Could you check a few things on this model? Use its own coordinates, in mm. Face numbers are marked on the shaded views. Give positions to 0.01 mm unless a question says otherwise; leave off trailing zeros. Loops run counter-clockwise (first coordinate to the right, second up) from the corner with the lowest first, then second, coordinate; pieces in that order, holes last. Notation, with made-up numbers: M 9,-23.5 L 39,-23.5 A15 ccw 39,0.5 Z; hole C -32.5,-4 d8. An arc over 180 degrees is marked long. Return JSON: item names as keys, results as strings. Group by question number.
1. If we section it at B-B (z = 25.5): Write out the boundary of the cut face in (x, y), plus the area to 3 significant figures.
2. If we mould it in two halves opening along Z, with no side actions, what happens to the marked faces 1, 2 and 3? For each: +Z half, -Z half, draft (parallel to the pull), parting line (faces both ways), or undercut.
3. If we section it at A-A (z = -31): Write out the boundary of the cut face in (x, y), plus the area to 3 significant figures.
4. For pin 1 (6 mm diameter, centred on x = -10, z = 38, fed in from -Y); pin 2 (8 mm diameter, centred on x = -10, y = -1.5, fed in from -Z); pin 3 (4 mm diameter, centred on x = -2.5, y = -7, fed in from -Z), each with a flat end and sliding along its axis, tell me the tip position at first contact or that it passes through.
5. Please list where these lines run through material, in increasing order: line 1 (Y direction, x = 1, z = 71); line 2 (X direction, y = 0.5, z = 16); line 3 (Z direction, x = 5.5, y = -9).
```python
from build123d import *

# Parameters (mm, degrees)
F0_R     = 17.3493533367
F1_DEPTH = 107.62834
F2_R     = 5.08
F3_R     = 5.08
F4_R     = 7.3657213081
F5_DEPTH = 42.52659
F6_R     = 9.8562945963
F7_DEPTH = 4.6773


# Not quite as in the source:
# - a fillet or chamfer that OpenCascade refuses, or shapes differently, is made with other operations: its cross-section is extruded or revolved along the edge and cut away or added


with BuildPart() as f1:
    # F0 (on Top) → F1 (new body)
    with BuildSketch(Plane.XY):
        Circle(F0_R)
    extrude(amount=F1_DEPTH)

    # F2
    f2_edges = [f1.edges().sort_by_distance(p)[0] for p in [
        (-17.349353, 0, 107.62834),
    ]]
    fillet(f2_edges, radius=F2_R)

    # F3
    f3_edges = [f1.edges().sort_by_distance(p)[0] for p in [
        (-17.349353, 0, 0),
    ]]
    fillet(f3_edges, radius=F3_R)

    # F4 (on Top) → F5 (join)
    with BuildSketch(Plane.XY):
        Circle(F4_R)
    extrude(amount=-F5_DEPTH)

    # F6 (on face) → F7 (join)
    with BuildSketch(Plane(origin=(0, 0, -42.52659), x_dir=(1, 0, 0), z_dir=(0, 0, -1))):
        Circle(F6_R)
    extrude(amount=F7_DEPTH)

    # F8: fillet of radius 5.08 on 1 edges, made by hand

    # F8_s1 → F8_t2 (revolve, cut)
    with BuildSketch(Plane.XZ):
        with BuildLine():
            ThreePointArc((9.8562945963, -42.52659), (8.2390682978, -45.8556533901), (4.7922810981, -47.20389))
            Line((4.7922810981, -47.20389), (9.8562945963, -47.20389))
            Line((9.8562945963, -47.20389), (9.8562945963, -42.52659))
        make_face()
    revolve(axis=Axis((0, 0, -47.20389), (0, 0, -1)), mode=Mode.SUBTRACT)


solid = f1.part
```
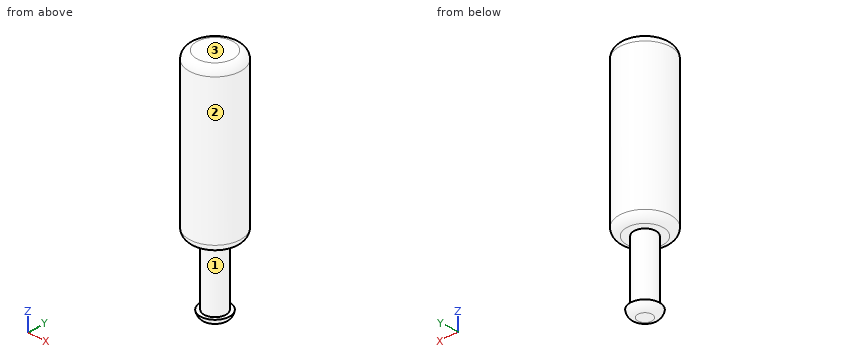
Answer:
{
 "1": {"outline": "C 0,0 d34.7", "area": "946 mm²"},
 "2": {"face 1": "undercut", "face 2": "draft", "face 3": "+Z half"},
 "3": {"outline": "C 0,0 d14.73", "area": "170 mm²"},
 "4": {"pin 1": "stops at y = -15.87", "pin 2": "stops at z = -47.03", "pin 3": "stops at z = -47.16"},
 "5": {"line 1": "y = -17.32 to 17.32", "line 2": "x = -17.34 to 17.34", "line 3": "z = 0 to 107.63"}
}
